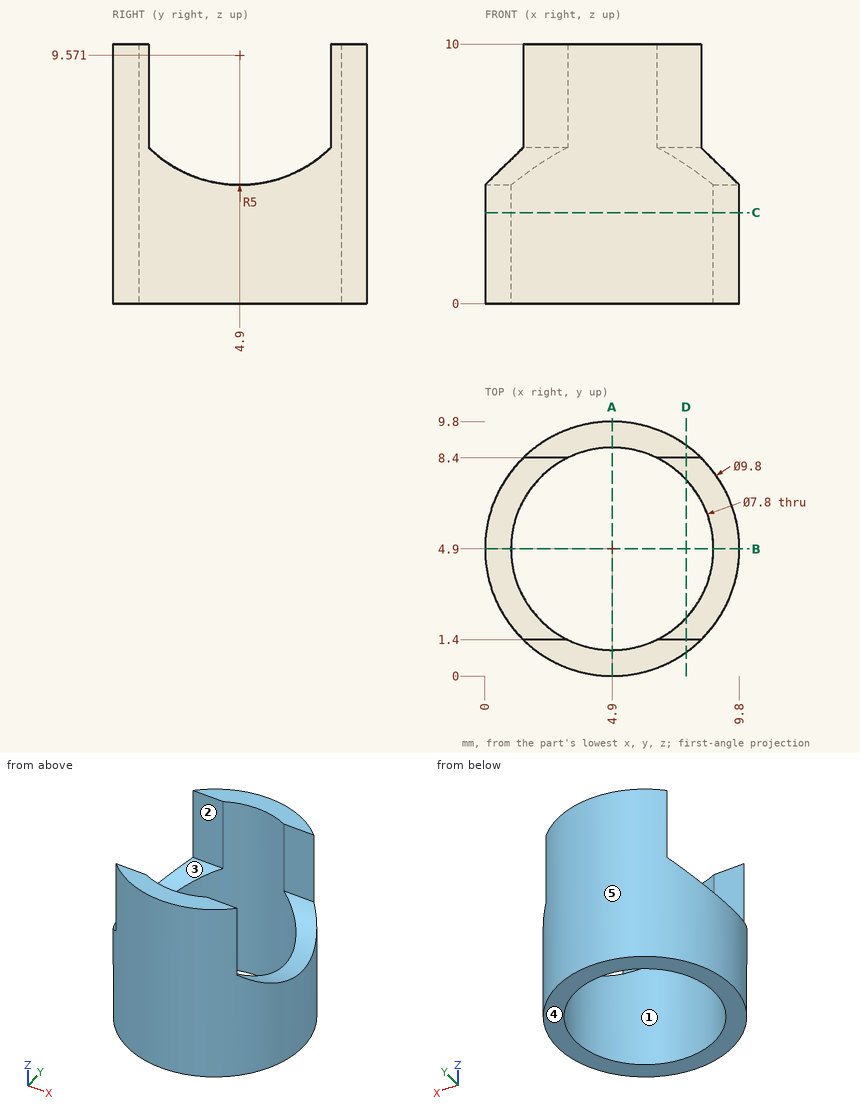
Geometry check sheet. Reference: drawing and pictorial views, mm from the part's lowest x, y, z. A direction names the side the tool comes from. Coordinates: 2 decimals unless noted, no trailing zeros. Loops run counter-clockwise (first coordinate to the right, second up) from the corner with the lowest first, then second, coordinate; pieces in that order, holes last. Notation, with made-up numbers: (-24.75, 78.5) - (-13.75, 78.5) arc R17 cw to (-13.75, 90.5) - close; hole circle Ø6 at (-33.5, 70.5). An arc over 180 degrees is marked (long way). Return JSON: item names as keys, results as strings.
1. Go/stop test with flat-tipped pins: pin 1 (0.5 mm diameter, centred on x = 2.5, z = 7, fed in from -Y); pin 2 (2 mm diameter, centred on x = 7, z = 2, fed in from +Y) (1 decimal); pin 3 (1.4 mm diameter, centred on x = 8, z = 7.5, fed in from -Y). Record where each tip stops, or that it passes through.
Established:
{"pin 1": "stops at y = 0.5", "pin 2": "stops at y = 9.7", "pin 3": "stops at y = 0.63"}
2. Mould release check, pull along Y, two halves, no side actions. Record for the marked faces 3, 4 and 5: +Y half, -Y half, draft (parallel to the pull), parting line (faces both ways), or undercut.
Established:
{"face 3": "undercut", "face 4": "draft", "face 5": "parting line"}
3. Section check C-C, the plane z = 3.5. Record the boundary of the cut face in (x, y).
Established:
{"outline": "circle Ø9.8 at (4.9, 4.9); hole circle Ø7.8 at (4.9, 4.9)"}
4. Section check A-A, the plane x = 4.9. Record the boundary of the cut face in (y, z).
Established:
{"outline": "(0, 0) - (1, 0) - (1, 10) - (0, 10) - close; (8.8, 0) - (9.8, 0) - (9.8, 10) - (8.8, 10) - close"}
5. Thickness scan on L1, parallel to Y at x = 4.9, z = 7; L2, parallel to Y at x = 8.5, z = 2.75 (1 decimal); L3, parallel to X at y = 3.25, z = 1.5. Record the ranges inside material, lowest first.
Established:
{"L1": "y = 0 to 1, 8.8 to 9.8", "L2": "y = 1.6 to 3.4, 6.4 to 8.2", "L3": "x = 0.29 to 1.37, 8.43 to 9.51"}
6. Tool access check on the marked faces 1 and 2. Record the directions out of +Z, -Z, +X, -X, +Y, -Y that give a thin tool (end or side, any length) a straight path to the whole face; none if there is none.
Established:
{"face 1": "+Z, -Z", "face 2": "+Z, +X, -X"}
7. Section check D-D, the plane x = 7.75. Record the boundary of the cut face in (y, z).
Established:
{"outline": "(0.91, 0) - (2.24, 0) - (2.24, 5.34) arc R5 cw to (1.4, 6) - (1.4, 10) - (0.91, 10) - close; (7.56, 0) - (8.89, 0) - (8.89, 10) - (8.4, 10) - (8.4, 6) arc R5 cw to (7.56, 5.34) - close"}
8. Section check B-B, the plane y = 4.9. Record the boundary of the cut face in (x, z).
Established:
{"outline": "(0, 0) - (1, 0) - (1, 4.57) - (0, 4.57) - close; (8.8, 0) - (9.8, 0) - (9.8, 4.57) - (8.8, 4.57) - close"}
